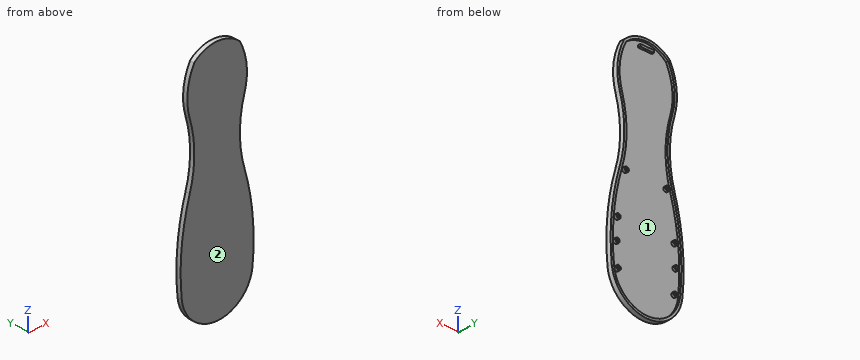
```python
from build123d import *

# Parameters (mm, degrees)
BOSS_EXTRUDE1_DEPTH = 3.175
CUT_EXTRUDE1_DEPTH  = 1.5875
SKETCH2_R           = 1.5875
SKETCH2_R_2         = 0.79375
SKETCH2_W           = 9.525
SKETCH2_H           = 1.5875
BOSS_EXTRUDE3_DEPTH = 1.5875


with BuildPart() as part:
    # Sketch1 → Boss-Extrude1 (new body)
    with BuildSketch(Plane(origin=(0, 0, 0), x_dir=(1, 0, 0), z_dir=(0, 1, 0))):
        with BuildLine():
            ThreePointArc((-24.608229426, 60.285411471), (0, 82.55), (24.608229426, 60.285411471))
            ThreePointArc((24.608229426, 60.285411471), (24.729538057, 29.875290817), (19.05, 0))
            ThreePointArc((19.05, 0), (15.875, -22.225), (19.05, -44.45))
            ThreePointArc((19.05, -44.45), (20.544089225, -60.633158922), (15.875, -76.2))
            ThreePointArc((15.875, -76.2), (0, -82.55), (-15.875, -76.2))
            ThreePointArc((-15.875, -76.2), (-20.544089225, -60.633158922), (-19.05, -44.45))
            ThreePointArc((-19.05, -44.45), (-15.875, -22.225), (-19.05, 0))
            ThreePointArc((-19.05, 0), (-24.729538057, 29.875290817), (-24.608229426, 60.285411471))
        make_face()
    extrude(amount=BOSS_EXTRUDE1_DEPTH)

    # Sketch3 → Cut-Extrude1 (cut)
    with BuildSketch(Plane(origin=(0, 3.175, 0), x_dir=(1, 0, 0), z_dir=(0, 1, 0))):
        with BuildLine():
            ThreePointArc((-17.526, -44.8945), (-18.977391367, -60.343827238), (-14.591091342, -75.228336673))
            ThreePointArc((-14.591091342, -75.228336673), (0, -80.9625), (14.591091342, -75.228336673))
            ThreePointArc((14.591091342, -75.228336673), (18.977391367, -60.343827238), (17.526, -44.8945))
            ThreePointArc((17.526, -44.8945), (14.2875, -22.225), (17.526, 0.4445))
            ThreePointArc((17.526, 0.4445), (23.148742676, 30.021037909), (23.028647132, 60.127057357))
            ThreePointArc((23.028647132, 60.127057357), (0, 80.9625), (-23.028647132, 60.127057357))
            ThreePointArc((-23.028647132, 60.127057357), (-23.148742676, 30.021037909), (-17.526, 0.4445))
            ThreePointArc((-17.526, 0.4445), (-14.2875, -22.225), (-17.526, -44.8945))
        make_face()
    extrude(amount=-CUT_EXTRUDE1_DEPTH, mode=Mode.SUBTRACT)

    # Sketch2 → Boss-Extrude3 (add)
    # profile 1 of 9: a face of its own
    with BuildSketch(Plane(origin=(0, 3.175, 0), x_dir=(1, 0, 0), z_dir=(0, 1, 0))):
        with Locations(Location((-19.845729426, 60.285411471, 0), (0, 0, 270))):
            Circle(SKETCH2_R)
        with Locations(Location((-19.845729426, 60.285411471, 0), (0, 0, 270))):
            Circle(SKETCH2_R_2, mode=Mode.SUBTRACT)
    # profile 2 of 9: a face of its own
    with BuildSketch(Plane(origin=(0, 3.175, 0), x_dir=(1, 0, 0), z_dir=(0, 1, 0))):
        with Locations(Location((-20.6375, 44.45, 0), (0, 0, 270))):
            Circle(SKETCH2_R)
        with Locations(Location((-20.6375, 44.45, 0), (0, 0, 270))):
            Circle(SKETCH2_R_2, mode=Mode.SUBTRACT)
    # profile 3 of 9: a face of its own
    with BuildSketch(Plane(origin=(0, 3.175, 0), x_dir=(1, 0, 0), z_dir=(0, 1, 0))):
        with Locations(Location((-19.967038057, 29.875290817, 0), (0, 0, 270))):
            Circle(SKETCH2_R)
        with Locations(Location((-19.967038057, 29.875290817, 0), (0, 0, 270))):
            Circle(SKETCH2_R_2, mode=Mode.SUBTRACT)
    # profile 4 of 9: a face of its own
    with BuildSketch(Plane(origin=(0, 3.175, 0), x_dir=(1, 0, 0), z_dir=(0, 1, 0))):
        with Locations(Location((-14.2875, 0, 0), (0, 0, 270))):
            Circle(SKETCH2_R)
        with Locations(Location((-14.2875, 0, 0), (0, 0, 270))):
            Circle(SKETCH2_R_2, mode=Mode.SUBTRACT)
    # profile 5 of 9: a face of its own
    with BuildSketch(Plane(origin=(0, 3.175, 0), x_dir=(1, 0, 0), z_dir=(0, 1, 0))):
        with Locations(Location((19.845729426, 60.285411471, 0), (0, 0, 270))):
            Circle(SKETCH2_R)
        with Locations(Location((19.845729426, 60.285411471, 0), (0, 0, 270))):
            Circle(SKETCH2_R_2, mode=Mode.SUBTRACT)
    # profile 6 of 9: a face of its own
    with BuildSketch(Plane(origin=(0, 3.175, 0), x_dir=(1, 0, 0), z_dir=(0, 1, 0))):
        with Locations(Location((20.6375, 44.45, 0), (0, 0, 270))):
            Circle(SKETCH2_R)
        with Locations(Location((20.6375, 44.45, 0), (0, 0, 270))):
            Circle(SKETCH2_R_2, mode=Mode.SUBTRACT)
    # profile 7 of 9: a face of its own
    with BuildSketch(Plane(origin=(0, 3.175, 0), x_dir=(1, 0, 0), z_dir=(0, 1, 0))):
        with Locations(Location((19.967038057, 29.875290817, 0), (0, 0, 270))):
            Circle(SKETCH2_R)
        with Locations(Location((19.967038057, 29.875290817, 0), (0, 0, 270))):
            Circle(SKETCH2_R_2, mode=Mode.SUBTRACT)
    # profile 8 of 9: a face of its own
    with BuildSketch(Plane(origin=(0, 3.175, 0), x_dir=(1, 0, 0), z_dir=(0, 1, 0))):
        with Locations(Location((14.2875, 0, 0), (0, 0, 270))):
            Circle(SKETCH2_R)
        with Locations(Location((14.2875, 0, 0), (0, 0, 270))):
            Circle(SKETCH2_R_2, mode=Mode.SUBTRACT)
    # profile 9 of 9: a face of its own
    with BuildSketch(Plane(origin=(0, 3.175, 0), x_dir=(1, 0, 0), z_dir=(0, 1, 0))):
        with Locations((0, -76.99375)):
            Rectangle(SKETCH2_W, SKETCH2_H)
    extrude(amount=-BOSS_EXTRUDE3_DEPTH)


solid = part.part
```
Geometry check sheet. Reference: the model listing, model coordinates, mm. Face numbers are marked on the shaded views. Coordinates: 2 decimals unless noted, no trailing zeros. Loops run counter-clockwise (first coordinate to the right, second up) from the corner with the lowest first, then second, coordinate; pieces in that order, holes last.
Item 1: Sectioned sample at C-C, the plane x = 2.5. Record the boundary of the cut face in (y, z) (1 decimal), then the cut area to 3 significant figures.
Item 2: Sectioned sample at B-B, the plane z = 70.5. Record the boundary of the cut face in (x, y) (1 decimal), then the cut area to 3 significant figures.
Item 3: Release check for a two-part mould opening along X. For the marked faces 1 and 2 record: released by +X, released by -X, zero draft, split by the parting line, or undercut.
Item 4: Thickness scan on line 1 (Y direction, x = -14, z = -22); line 2 (X direction, y = 0.5, z = 53); line 3 (X direction, y = 3, z = -20). Record the ranges inside material, lowest first.
Item 5: Go/stop test with flat-tipped pins: pin 1 Ø1.4 at (x, z) = (20.64, -44.45) entering from +Y; pin 2 Ø1.7 at (x, z) = (-14.5, -0.5) entering from +Y (3 decimals); pin 3 Ø1.7 at (x, y) = (-0.5, 2.5) entering from -Z; pin 4 Ø1.3 at (y, z) = (2, 77) entering from +X. Record where each tip stops, or that it passes through.
Check result:
1. outline: (0, -82.4) - (3.2, -82.4) - (3.2, -80.8) - (1.6, -80.8) - (1.6, 76.2) - (3.2, 76.2) - (3.2, 77.8) - (1.6, 77.8) - (1.6, 80.8) - (3.2, 80.8) - (3.2, 82.4) - (0, 82.4) - close
1. area: 269 mm2
2. outline: (-18.4, 0) - (18.4, 0) - (18.4, 3.2) - (16.7, 3.2) - (16.7, 1.6) - (-16.7, 1.6) - (-16.7, 3.2) - (-18.4, 3.2) - close
2. area: 63.6 mm2
3. face 1: undercut
3. face 2: zero draft
4. line 1: y = 0 to 1.59
4. line 2: x = -20.62 to 20.62
4. line 3: x = -23.51 to -21.9, 21.9 to 23.51
5. pin 1: stops at y = 1.59
5. pin 2: stops at y = 3.175
5. pin 3: stops at z = -82.55
5. pin 4: stops at x = 15.72
